Read the model definition and answer for the solid it produces. Units are mm, in the model's axes. Coordinates: 2 decimals unless noted, no trailing zeros. Loops run counter-clockwise (first coordinate to the right, second up) from the corner with the lowest first, then second, coordinate; pieces in that order, holes last. Notation, with made-up numbers: (-3, 88) -> (30, 88) arc R28 cw to (30, 127) -> close; hole circle Ø10 at (-12.75, -35.75). An arc over 180 degrees is marked (long way). Answer in a Markdown table with one row per item.
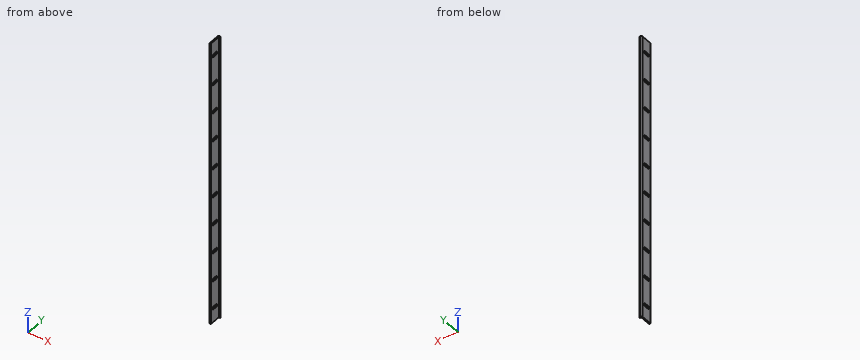
```python
from build123d import *

# Parameters (mm, degrees)
BOSS_EXTRUDE1_DEPTH = 500
FILLET1_R           = 0.50329666
FILLET2_R           = 0.50398302
FILLET3_R           = 0.30157619
FILLET4_R           = 0.30157551
CUT_EXTRUDE1_DEPTH  = 2.375
LPATTERN1_COUNT     = 10
LPATTERN1_PITCH     = 50


with BuildPart() as part:
    # Sketch1 → Boss-Extrude1 (new body)
    with BuildSketch(Plane.XY):
        with BuildLine():
            Line((0, 20.330194912), (2.019589054, 22.349783966))
            ThreePointArc((2.019589054, 22.349783966), (2.375, 22.497), (2.730410946, 22.349783966))
            Line((2.730410946, 22.349783966), (4.75, 20.330194912))
            Line((4.75, 20.330194912), (4.75, 19.5291))
            Line((4.75, 19.5291), (2.375, 19.5291))
            Line((2.375, 19.5291), (2.375, 0))
            Line((2.375, 0), (0, 0))
            Line((0, 0), (0, 20.330194912))
        make_face()
    extrude(amount=BOSS_EXTRUDE1_DEPTH)

    # Fillet1
    fillet1_edges = [part.edges().sort_by_distance(p)[0] for p in [
        (0, 20.330194912, 250),
    ]]
    fillet(fillet1_edges, radius=FILLET1_R)

    # Fillet2
    fillet2_edges = [part.edges().sort_by_distance(p)[0] for p in [
        (4.75, 20.330194912, 250),
    ]]
    fillet(fillet2_edges, radius=FILLET2_R)

    # Fillet3
    fillet3_edges = [part.edges().sort_by_distance(p)[0] for p in [
        (4.75, 19.5291, 250),
    ]]
    fillet(fillet3_edges, radius=FILLET3_R)

    # Fillet4
    fillet4_edges = [part.edges().sort_by_distance(p)[0] for p in [
        (2.375, 0, 250),
        (0, 0, 250),
    ]]
    fillet(fillet4_edges, radius=FILLET4_R)

    # Sketch2 → Cut-Extrude1 (cut)
    with BuildSketch(Plane.ZY):
        with BuildLine():
            Line((27.65, 13.1043), (27.65, 6.4043))
            ThreePointArc((27.65, 6.4043), (25, 3.7543), (22.35, 6.4043))
            Line((22.35, 6.4043), (22.35, 13.1043))
            ThreePointArc((22.35, 13.1043), (25, 15.7543), (27.65, 13.1043))
        make_face()
    cut_extrude1 = extrude(amount=-CUT_EXTRUDE1_DEPTH, mode=Mode.SUBTRACT)

    # LPattern1: Cut-Extrude1 ×10
    with Locations(*[(0, 0, i * LPATTERN1_PITCH) for i in range(1, LPATTERN1_COUNT)]):
        add(cut_extrude1, mode=Mode.SUBTRACT)


solid = part.part
```
1. Find the intervals of material crossed by probe 1 along X at (y, z) = (3.5, 405) (3 decimals); probe 2 along Y at (x, z) = (2.25, 252); probe 3 along Y at (x, z) = (2.65, 426), in increasing order.
A:
| item | result |
|---|---|
| probe 1 | x = 0 to 2.375 |
| probe 2 | y = 0.06 to 22.48 |
| probe 3 | y = 19.53 to 22.42 |
2. A cutting plane is placed at A-A on z = 152.5. Give the vertices of the cut face in (x, y) (3 decimals).
A:
| item | result |
|---|---|
| outline | (0, 0.302) arc R0.302 ccw to (0.302, 0) -> (2.073, 0) arc R0.302 ccw to (2.375, 0.302) -> (2.375, 19.529) -> (4.448, 19.529) arc R0.302 ccw to (4.75, 19.831) -> (4.75, 20.121) arc R0.504 ccw to (4.602, 20.478) -> (2.73, 22.35) arc R0.503 ccw to (2.02, 22.35) -> (0.147, 20.478) arc R0.503 ccw to (0, 20.122) -> close |
3. Given pin 1 Ø2.5 at (x, y) = (1, 11) entering from -Z; pin 2 Ø1 at (y, z) = (11, 285.5) entering from +X (3 decimals), each flat-ended and moving along its own axis, determine where each tip first touches the part or whether it passes through.
A:
| item | result |
|---|---|
| pin 1 | stops at z = 0 |
| pin 2 | stops at x = 2.375 |
